Geometry: final body of the model. Coordinates: model frame, mm. A direction names the side the tool comes from. Give positions to 0.01 mm unless a question says otherwise; leave off trailing zeros. Order: outer loops, then holes, each group sorted by start corner. A loop starts at its lowest first (then second) coordinate and runs counter-clockwise, first axis right, second up. Notation, with made-up numbers: (72.5, 88.25) -> (116.5, 88.25) arc R26 cw to (116.5, 117.25) -> close; hole circle Ø5 at (57, 32.5). An arc over 180 degrees is marked (long way). Answer in a Markdown table with one row per item. Add a question column.
Q1. Set-up query: faces 4 (the face through (42, 6.75, -3)), 5 (the face through (44, 62, 3)). Return all of +Z, -Z, +X, -X, +Y, -Y with unobstructed straight access to the full face (end or side cutting, diameter ignored); none if empty.
Q2. Pull-direction query (X, two-part tool) for faces 1 (the face through (0, 32, -2)), 2 (the face through (44, 65, -2)), 3 (the face through (39.5, 9.7, 0)); classes: +X half, -X half, draft (parallel to the pull), parting line (faces both ways), or undercut.
Q3. Cut plane A-A on z = -5. Return the cut outline in (x, y).
Q4. Line query: line 1 along Y through (x, z) = (20, -4.75); line 2 along X through (y, z) = (23.5, -2.5); line 3 along X through (y, z) = (39, 2.25). Output: solid intervals per line, ascending. Write a range as from..to.
Q5. Contact query for flat-ended pins moving along their axis: P1, Ø2, axis at x = 11, z = -3, coming from the -Y side; P2, Ø10, axis at x = 28, y = 17.5, coming from the +Z side. Output: stop coordinate, or through.
from build123d import *

# Parameters (mm, degrees)
SKETCH_W     = 90
SKETCH_H     = 65
PAD_DEPTH    = 10
SKETCH004_W  = 71
SKETCH004_H  = 51
POCKET_DEPTH = 7
SKETCH003_W  = 71
SKETCH003_H  = 51
SKETCH001_W  = 65
SKETCH001_H  = 45


with BuildPart() as part:
    # Sketch → Pad (new body)
    with BuildSketch(Plane.XY.offset(3)):
        with Locations((45, 32.5)):
            Rectangle(SKETCH_W, SKETCH_H)
    extrude(amount=-PAD_DEPTH)

    # Sketch004 → Pocket (cut)
    with BuildSketch(Plane.XY):
        with Locations((42.25, 32.25)):
            Rectangle(SKETCH004_W, SKETCH004_H)
    extrude(amount=-POCKET_DEPTH, mode=Mode.SUBTRACT)

    # Sketch003 → SubtractiveLoft section 0
    with BuildSketch(Plane.XY.offset(3)):
        with Locations((42.5, 32.5)):
            Rectangle(SKETCH003_W, SKETCH003_H)
    # Sketch001 → SubtractiveLoft section 1
    with BuildSketch(Plane.XY):
        with Locations((42.5, 32.5)):
            Rectangle(SKETCH001_W, SKETCH001_H)
    loft(mode=Mode.SUBTRACT)


solid = part.part
Completed:
| question | item | result |
|---|---|---|
| 1 | face 4 | -Z |
| 1 | face 5 | +Z, +X, -X, +Y, -Y |
| 2 | face 1 | -X half |
| 2 | face 2 | draft |
| 2 | face 3 | undercut |
| 3 | outline | (0, 0) -> (90, 0) -> (90, 65) -> (0, 65) -> close; hole (6.75, 6.75) -> (77.75, 6.75) -> (77.75, 57.75) -> (6.75, 57.75) -> close |
| 4 | line 1 | y = 0..6.75, 57.75..65 |
| 4 | line 2 | x = 0..6.75, 77.75..90 |
| 4 | line 3 | x = 0..7.75, 77.25..90 |
| 5 | P1 | stops at y = 0 |
| 5 | P2 | passes through |
